```python
from build123d import *

# Parameters (mm, degrees)
SKETCH2_W           = 136.525
SKETCH2_H           = 787.4
BOSS_EXTRUDE1_DEPTH = 88.9
SKETCH4_W           = 85.725
SKETCH4_H           = 44.45
BOSS_EXTRUDE2_DEPTH = 25.4
SKETCH5_W           = 25.4
SKETCH5_H           = 82.55
CUT_EXTRUDE1_DEPTH  = 50.8
SKETCH6_W           = 15.875
SKETCH6_H           = 69.85
SKETCH6_H_2         = 88.9
CUT_EXTRUDE2_DEPTH  = 50.8
SKETCH7_R           = 4.7625
CUT_EXTRUDE3_DEPTH  = 44.45
SKETCH7_3_R         = 14.2875
CUT_EXTRUDE4_DEPTH  = 12.7
SKETCH7_4_R         = 6.35
CUT_EXTRUDE5_DEPTH  = 450.652194062


with BuildPart() as part:
    # Sketch2 → Boss-Extrude1 (new body)
    with BuildSketch(Plane.XY):
        Rectangle(SKETCH2_W, SKETCH2_H)
    extrude(amount=BOSS_EXTRUDE1_DEPTH)

    # Sketch4 → Boss-Extrude2 (add)
    with BuildSketch(Plane(origin=(0, 393.7, 0), x_dir=(1, 0, 0), z_dir=(0, 1, 0))):
        with Locations((0, -50.8)):
            Rectangle(SKETCH4_W, SKETCH4_H)
    extrude(amount=BOSS_EXTRUDE2_DEPTH)

    # Sketch5 → Cut-Extrude1 (cut)
    with BuildSketch(Plane.ZY.offset(68.2625)):
        with Locations((26.9875, -212.725)):
            Rectangle(SKETCH5_W, SKETCH5_H)
    extrude(amount=-CUT_EXTRUDE1_DEPTH, mode=Mode.SUBTRACT)

    # Sketch6 → Cut-Extrude2 (cut)
    with BuildSketch(Plane.XY.offset(88.9)):
        with Locations((46.0375, 339.725)):
            Rectangle(SKETCH6_W, SKETCH6_H)
        with Locations((46.0375, -212.725)):
            Rectangle(SKETCH6_W, SKETCH6_H_2)
    extrude(amount=-CUT_EXTRUDE2_DEPTH, mode=Mode.SUBTRACT)

    # Sketch7 → Cut-Extrude3 (cut)
    with BuildSketch(Plane(origin=(68.2625, 0, 0), x_dir=(0, 0, -1), z_dir=(1, 0, 0))):
        with Locations(Location((-63.5, -188.9125, 0), (0, 0, 90))):
            Circle(SKETCH7_R)
        with Locations(Location((-63.5, -236.5375, 0), (0, 0, 90))):
            Circle(SKETCH7_R)
        with Locations(Location((-63.5, 315.9125, 0), (0, 0, 90))):
            Circle(SKETCH7_R)
        with Locations(Location((-63.5, 363.5375, 0), (0, 0, 90))):
            Circle(SKETCH7_R)
    extrude(amount=-CUT_EXTRUDE3_DEPTH, mode=Mode.SUBTRACT)

    # Sketch7_3 → Cut-Extrude4 (cut)
    with BuildSketch(Plane(origin=(68.2625, 0, 0), x_dir=(0, 0, -1), z_dir=(1, 0, 0))):
        with Locations(Location((-26.9875, -212.725, 0), (0, 0, 90))):
            Circle(SKETCH7_3_R)
    extrude(amount=-CUT_EXTRUDE4_DEPTH, mode=Mode.SUBTRACT)

    # Sketch7_4 → Cut-Extrude5 (cut, through all)
    with BuildSketch(Plane(origin=(68.2625, 0, 0), x_dir=(0, 0, -1), z_dir=(1, 0, 0))):
        with Locations(Location((-26.9875, -212.725, 0), (0, 0, 90))):
            Circle(SKETCH7_4_R)
    extrude(amount=-CUT_EXTRUDE5_DEPTH, mode=Mode.SUBTRACT)


solid = part.part
```
Work out the finished part from the listing and answer in its coordinate system (mm). A direction names the side the tool comes from. Give positions to 0.01 mm unless a question says otherwise; leave off trailing zeros. One line per question, with ' | ' between items. Start each with the question number.
1) Straight lines are drawn through the part: L1, parallel to Y at x = 34, z = 63; L2, parallel to Z at x = -23, y = -215.5; L3, parallel to Y at x = 55.5, z = 27. For each, find the intervals that lie inside material, in ascending order.
2) This flat-tipped pin is pushed along its axis until it touches: pin 1 (14.5 mm diameter, centred on y = -212.72, z = 26.99, fed in from -X). Where does it stop, or does it pass through?
3) For faces 4 (the face through (38.1, 339, 64)), 5 (the face through (-1, 406, 73.025)), 6 (the face through (42.862, 406, 51)), 7 (the face through (-17.463, -212, 35)), determine the directions among +Z, -Z, +X, -X, +Y, -Y from which every point of the face is accessible in a straight line to the end or side of a thin tool.
4) Determine the mould class of faces 1 (the face through (-1, 393.7, 24)), 2 (the face through (62.001, -199.097, 31.279)), 3 (the face through (46, 340, 38.1)) for opening direction Z: +Z half, -Z half, draft (parallel to the pull), parting line (faces both ways), or undercut.
Resolved:
1) L1: -393.7 to -241.27, -231.8 to -193.65, -184.18 to 311.18, 320.65 to 358.8, 368.27 to 419.1 | L2: 0 to 14.29, 39.69 to 88.9 | L3: -393.7 to -219.07, -206.38 to 393.7
2) pin 1: x = -17.46
3) face 4: +Z | face 5: +Z, +X, -X, +Y | face 6: +Z, -Z, +X, +Y | face 7: -X
4) face 1: draft | face 2: undercut | face 3: +Z half
